```python
from build123d import *

# Parameters (mm, degrees)
SKETCH1_W           = 55
SKETCH1_H           = 12.7
BOSS_EXTRUDE1_DEPTH = 10
CUT_EXTRUDE1_DEPTH  = 32.898902802
SKETCH6_W           = 8.1
SKETCH6_H           = 3.1
SKETCH6_H_2         = 4
SKETCH7_R           = 1.75
CUT_EXTRUDE2_DEPTH  = 6.5
SKETCH8_R           = 3.25
CUT_EXTRUDE3_DEPTH  = 3
FILLET1_R           = 1


with BuildPart() as part:
    # Sketch1 → Boss-Extrude1 (new body)
    with BuildSketch(Plane.XY):
        Rectangle(SKETCH1_W, SKETCH1_H)
    extrude(amount=BOSS_EXTRUDE1_DEPTH)

    # Sketch2 → Cut-Extrude1 (cut, through all)
    with BuildSketch(Plane(origin=(0, 6.35, 0), x_dir=(1, 0, 0), z_dir=(0, 1, 0))):
        with BuildLine():
            Line((5.338539126, 0), (-5.338539126, 0))
            ThreePointArc((-5.338539126, 0), (0, -3), (5.338539126, 0))
        make_face()
        with BuildLine():
            Line((-17.062940163, 0), (-25.937059837, 0))
            ThreePointArc((-25.937059837, 0), (-21.5, -2.25), (-17.062940163, 0))
        make_face()
    extrude(amount=-CUT_EXTRUDE1_DEPTH, mode=Mode.SUBTRACT)

    # Sketch6 → Cut-Revolve1 (revolve, cut)
    with BuildSketch(Plane(origin=(0, 0, -3.25), x_dir=(-1, 0, 0), z_dir=(0, 0, -1))):
        with Locations((4.05, 4.8)):
            Rectangle(SKETCH6_W, SKETCH6_H)
        with Locations((4.05, -4.35)):
            Rectangle(SKETCH6_W, SKETCH6_H_2)
    revolve(axis=Axis((0, -6.35, -3.25), (0, 1, 0)), mode=Mode.SUBTRACT)

    # Sketch7 → Cut-Extrude2 (cut)
    with BuildSketch(Plane(origin=(0, 0, 0), x_dir=(-1, 0, 0), z_dir=(0, 0, -1))):
        with Locations((12.5, 0)):
            Circle(SKETCH7_R)
        with Locations((-12.5, 0)):
            Circle(SKETCH7_R)
    extrude(amount=-CUT_EXTRUDE2_DEPTH, mode=Mode.SUBTRACT)

    # Sketch8 → Cut-Extrude3 (cut)
    with BuildSketch(Plane.XY.offset(10)):
        with Locations((-12.5, 0)):
            Circle(SKETCH8_R)
        with Locations((12.5, 0)):
            Circle(SKETCH8_R)
    extrude(amount=-CUT_EXTRUDE3_DEPTH, mode=Mode.SUBTRACT)

    # Fillet1
    fillet1_edges = [part.edges().sort_by_distance(p)[0] for p in [
        (-27.5, 6.35, 5),
        (27.5, 6.35, 5),
        (27.5, -6.35, 5),
        (-27.5, -6.35, 5),
    ]]
    fillet(fillet1_edges, radius=FILLET1_R)


solid = part.part
```
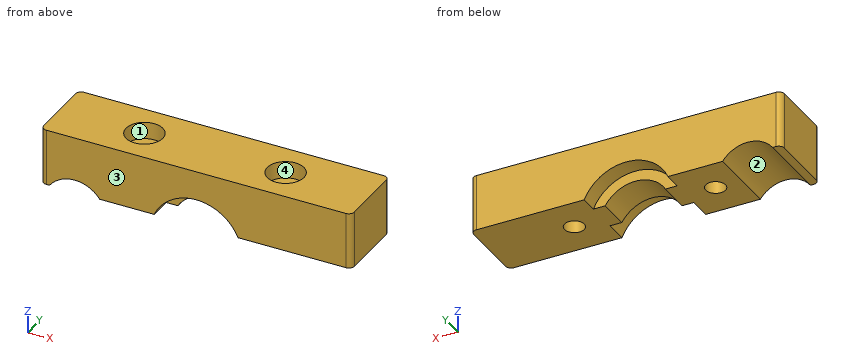
Work out the finished part from the listing and answer in its coordinate system (mm). Face numbers are marked on the shaded views. Coordinates: 2 decimals unless noted, no trailing zeros. Loops run counter-clockwise (first coordinate to the right, second up) from the corner with the lowest first, then second, coordinate; pieces in that order, holes last. Notation, with made-up numbers: (69.25, 28) - (92.25, 28) arc R19 ccw to (92.25, 46) - close; hole circle Ø1 at (23, 40.5). An arc over 180 degrees is marked (long way). Use a Markdown table: item, result.
Item 1: Given pin 1 Ø3 at (x, y) = (12.5, 0) entering from +Z; pin 2 Ø2.5 at (x, z) = (-2, 2) entering from +Y, each flat-ended and moving along its own axis, determine where each tip first touches the part or whether it passes through.
Evaluation:
| item | result |
|---|---|
| pin 1 | stops at z = 7 |
| pin 2 | stops at y = 3.25 |
Item 2: Find section D-D, the plane x = -12.5. Determine the outline of the cut face in (y, z), and give its area (4 significant figures).
Evaluation:
| item | result |
|---|---|
| outline | (-6.35, 0) - (-1.75, 0) - (-1.75, 6.5) - (1.75, 6.5) - (1.75, 0) - (6.35, 0) - (6.35, 10) - (3.25, 10) - (3.25, 7) - (-3.25, 7) - (-3.25, 10) - (-6.35, 10) - close |
| area | 84.75 mm2 |
Item 3: Find section A-A, the plane y = -4.25. Determine the outline of the cut face in (x, z), and give its area (3 significant figures).
Evaluation:
| item | result |
|---|---|
| outline | (-27.5, 0) - (-25.94, 0) arc R5.5 cw to (-17.06, 0) - (-7.42, 0) arc R8.1 cw to (7.42, 0) - (27.5, 0) - (27.5, 10) - (-27.5, 10) - close |
| area | 484 mm2 |
Item 4: Find section C-C, the plane z = 5.5. Determine the outline of the cut face in (x, y).
Evaluation:
| item | result |
|---|---|
| outline | (-27.5, -5.35) arc R1 ccw to (-26.5, -6.35) - (26.5, -6.35) arc R1 ccw to (27.5, -5.35) - (27.5, 5.35) arc R1 ccw to (26.5, 6.35) - (-26.5, 6.35) arc R1 ccw to (-27.5, 5.35) - close; hole circle Ø3.5 at (-12.5, 0); hole circle Ø3.5 at (12.5, 0) |
Item 5: The mould has two halves that part along Y. Classify the marked faces 1, 2, 3 and 4: +Y half, -Y half, draft (parallel to the pull), parting line (faces both ways), or undercut.
Evaluation:
| item | result |
|---|---|
| face 1 | undercut |
| face 2 | draft |
| face 3 | -Y half |
| face 4 | undercut |
Item 6: Consider probe 1 along Y at (x, z) = (12.5, 5); probe 2 along X at (y, z) = (-0.25, 1.75); probe 3 along X at (y, z) = (-2.5, 9.25). Determine where each line is inside the solid, lowest interval first. Write a range as from..to.
Evaluation:
| item | result |
|---|---|
| probe 1 | y = -6.35..-1.75, 1.75..6.35 |
| probe 2 | x = -27.5..-23.79, -19.21..-14.23, -10.77..-3.75, 3.75..10.77, 14.23..27.5 |
| probe 3 | x = -27.5..-14.58, -10.42..10.42, 14.58..27.5 |
Item 7: Find section B-B, the plane z = 1. Determine the outline of the cut face in (x, y), and give its area (3 significant figures).
Evaluation:
| item | result |
|---|---|
| outline | (-27.5, -5.35) arc R1 ccw to (-26.5, -6.35) - (-24.99, -6.35) - (-24.99, 6.35) - (-26.5, 6.35) arc R1 ccw to (-27.5, 5.35) - close; (-18.01, -6.35) - (-6.9, -6.35) - (-6.9, -2.35) - (-4.58, -2.35) - (-4.58, 3.25) - (-6.9, 3.25) - (-6.9, 6.35) - (-18.01, 6.35) - close; (4.58, -2.35) - (6.9, -2.35) - (6.9, -6.35) - (26.5, -6.35) arc R1 ccw to (27.5, -5.35) - (27.5, 5.35) arc R1 ccw to (26.5, 6.35) - (6.9, 6.35) - (6.9, 3.25) - (4.58, 3.25) - close; hole circle Ø3.5 at (-12.5, 0); hole circle Ø3.5 at (12.5, 0) |
| area | 440 mm2 |
